Part model, mm, in its own coordinate system. A direction names the side the tool comes from. Round coordinates to 2 decimals unless told otherwise and drop trailing zeros. Loops run counter-clockwise (first coordinate to the right, second up) from the corner with the lowest first, then second, coordinate; pieces in that order, holes last.
(1) Cut at A-A on x = 0. List the corners of the cut face in (y, z), then the cut area to 3 significant figures.
(2) Tool access for faces 1 (the face through (2.7, 4.001, 0.5)), 2 (the face through (2.376, 3, 0)): list every direction of +Z, -Z, +X, -X, +Y, -Y with a clear straight run to the whole face (end or side of a thin tool).
(3) Cut at C-C on x = 0.75. List the corners of the cut face in (y, z), then the cut area to 3 significant figures.
(4) Mould opens along Z. For faces 3 (the face through (0, 3, -4.75)), 4 (the face through (0, 3, 4.75)), 5 (the face through (0, 0, 0)), 6 (the face through (0, 2, -5.75)) say: +Z half, -Z half, draft (parallel to the pull), parting line (faces both ways), or undercut.
(5) Flat gauge pin, fed straight in: pin 1 (0.9 mm diameter, centred on y = 2.5, z = 1, fed in from -X). Where does the tip first touch, or does it go through?
(6) Cut at D-D on y = 2.2. List the corners of the cut face in (x, z), then the cut area to 3 significant figures.
(7) Probe probe 1 along Z at (x, y) = (0, 0.8); probe 2 along Z at (x, y) = (1.75, 3.3); probe 3 along Y at (x, z) = (1.75, 1). List the from-to ranges inside material, lowest first.
(8) Cut at B-B on z = -2.5. List the corners of the cut face in (x, y), then the cut area to 3 significant figures.
Autodesk Inventor part; units mm, degrees
ref_plane "YZ Plane" through (0, 0, 0) normal (1, 0, 0) x (0, 1, 0)
ref_plane "XZ Plane" through (0, 0, 0) normal (0, 1, 0) x (-1, 0, 0)
ref_plane "XY Plane" through (0, 0, 0) normal (0, 0, 1) x (1, 0, 0)
sketch "Sketch1" plane through (0, 0, 0) normal (0, 1, 0) x (-1, 0, 0)
  line L0 (3.07, 5.7495) -> (-3.07, 5.7495)
  line L1 (-3.07, 5.7495) -> (-3.07, -5.7495)
  line L2 (-3.07, -5.7495) -> (3.07, -5.7495)
  line L3 (3.07, -5.7495) -> (3.07, 5.7495)
  line L4 (3.07, 0) -> (-3.07, 0) construction
  line L5 (0, 5.7495) -> (0, -5.7495) construction
  point P0 (0, 0)
  point P1 (0, 0)
  point P2 (0, 0)
  point P3 (0, 0)
  dimension "d0" = 6.14
  dimension "d1" = 11.499
extrude "Extrusion1" add sketch "Sketch1" along normal blind 4.001
sketch "Sketch2" plane through (0, 4.001, 0) normal (0, 1, 0) x (1, 0, 0)
  line L0 (-7.624, -4.7495) -> (2.376, -4.7495)
  line L1 (2.376, -4.7495) -> (2.376, 4.7495)
  line L2 (2.376, 4.7495) -> (-7.624, 4.7495)
  line L3 (-7.624, 4.7495) -> (-7.624, -4.7495)
  line L4 (-5, 0) -> (5, 0) construction
  line L5 (0, -4.7495) -> (0, 4.7495) construction
  point P0 (0, 0)
  point P1 (0, 0)
  point P2 (0, 0)
  dimension "d4" = 9.499
  dimension "d5" = 10
extrude "Extrusion2" cut sketch "Sketch2" against normal blind 3.001
sketch "Sketch3" plane through (0, 0, 0) normal (0, -1, 0) x (1, 0, 0)
  circle A0 centre (0, -2.356) radius 0.5
  line L0 (-3.07, 4.7495) -> (-3.07, -4.7495) construction
  line L1 (-3.07, 0) -> (3.07, 0) construction
  line L2 (3.07, 5.7495) -> (3.07, -5.7495) construction
  circle A1 centre (0, 2.356) radius 0.5
  point P0 (0, 0)
  dimension "d8" = 1
hole "Hole1" at (0, 0, -2.356) at (0, 0, 2.356) direction (0, 1, 0) diameter 1 end through all
properties part number "LDR_Shield"
Final values:
1. outline: (0, -5.75) - (4, -5.75) - (4, -4.75) - (1, -4.75) - (1, -2.86) - (0, -2.86) - close; (0, -1.86) - (1, -1.86) - (1, 1.86) - (0, 1.86) - close; (0, 2.86) - (1, 2.86) - (1, 4.75) - (4, 4.75) - (4, 5.75) - (0, 5.75) - close
1. area: 15.5 mm2
2. face 1: +Z, -Z, +X, -X, +Y
2. face 2: -X, +Y
3. outline: (0, -5.75) - (4, -5.75) - (4, -4.75) - (1, -4.75) - (1, 4.75) - (4, 4.75) - (4, 5.75) - (0, 5.75) - close
3. area: 17.5 mm2
4. face 3: undercut
4. face 4: undercut
4. face 5: draft
4. face 6: -Z half
5. pin 1: stops at x = 2.38
6. outline: (-3.07, -5.75) - (3.07, -5.75) - (3.07, 5.75) - (-3.07, 5.75) - (-3.07, 4.75) - (2.38, 4.75) - (2.38, -4.75) - (-3.07, -4.75) - close
6. area: 18.9 mm2
7. probe 1: z = -5.75 to -2.86, -1.86 to 1.86, 2.86 to 5.75
7. probe 2: z = -5.75 to -4.75, 4.75 to 5.75
7. probe 3: y = 0 to 1
8. outline: (-3.07, 0) - (-0.48, 0) - (-0.48, 1) - (-3.07, 1) - close; (0.48, 0) - (3.07, 0) - (3.07, 4) - (2.38, 4) - (2.38, 1) - (0.48, 1) - close
8. area: 7.27 mm2
